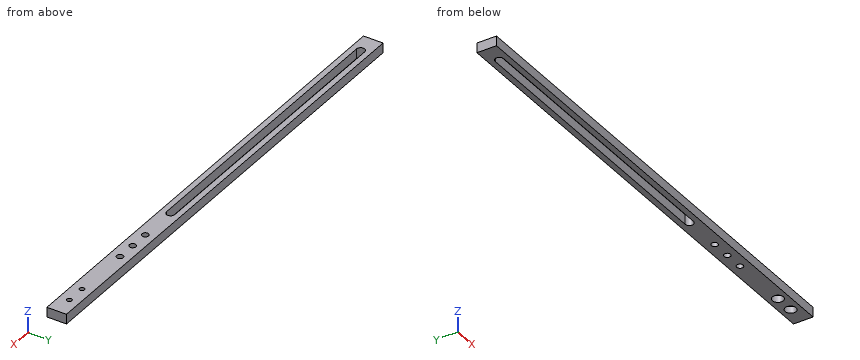
from build123d import *

# Parameters (mm, degrees)
SKETCH_1_W          = 250
SKETCH_1_H          = 10
EXTRUDE_1_DEPTH     = 5
CUT_EXTRUDE_1_DEPTH = 5
SKETCH_3_R          = 1.25
CUT_EXTRUDE_2_DEPTH = 5
SKETCH_4_R          = 2.8
CUT_EXTRUDE_3_DEPTH = 3.5
SKETCH_5_R          = 1.65
CUT_EXTRUDE_4_DEPTH = 10


with BuildPart() as part:
    # Эскиз1 → Бобышка-Вытянуть1 (new body)
    with BuildSketch(Plane.XY):
        Rectangle(SKETCH_1_W, SKETCH_1_H)
    extrude(amount=EXTRUDE_1_DEPTH)

    # Эскиз2 → Вырез-Вытянуть1 (cut)
    with BuildSketch(Plane(origin=(0, 0, 0), x_dir=(-1, 0, 0), z_dir=(0, 0, -1))):
        with BuildLine():
            Line((-35, 2.1), (115, 2.1))
            ThreePointArc((115, 2.1), (117.1, 0), (115, -2.1))
            Line((115, -2.1), (-35, -2.1))
            ThreePointArc((-35, -2.1), (-37.1, 0), (-35, 2.1))
        make_face()
    extrude(amount=-CUT_EXTRUDE_1_DEPTH, mode=Mode.SUBTRACT)

    # Эскиз3 → Вырез-Вытянуть2 (cut)
    with BuildSketch(Plane(origin=(0, 0, 0), x_dir=(-1, 0, 0), z_dir=(0, 0, -1))):
        with Locations((-115, 0)):
            Circle(SKETCH_3_R)
        with Locations((-105, 0)):
            Circle(SKETCH_3_R)
    extrude(amount=-CUT_EXTRUDE_2_DEPTH, mode=Mode.SUBTRACT)

    # Эскиз4 → Вырез-Вытянуть3 (cut)
    with BuildSketch(Plane(origin=(0, 0, 0), x_dir=(-1, 0, 0), z_dir=(0, 0, -1))):
        with Locations((-115, 0)):
            Circle(SKETCH_4_R)
        with Locations((-105, 0)):
            Circle(SKETCH_4_R)
    extrude(amount=-CUT_EXTRUDE_3_DEPTH, mode=Mode.SUBTRACT)

    # Эскиз5 → Вырез-Вытянуть4 (cut)
    with BuildSketch(Plane(origin=(0, 0, 0), x_dir=(-1, 0, 0), z_dir=(0, 0, -1))):
        with Locations((-75, 0)):
            Circle(SKETCH_5_R)
        with Locations((-65, 0)):
            Circle(SKETCH_5_R)
        with Locations((-55, 0)):
            Circle(SKETCH_5_R)
    extrude(amount=-CUT_EXTRUDE_4_DEPTH, mode=Mode.SUBTRACT)


solid = part.part
Read the model definition and answer for the solid it produces. Units are mm, in the model's axes. Give positions to 0.01 mm unless a question says otherwise; leave off trailing zeros. Loops run counter-clockwise (first coordinate to the right, second up) from the corner with the lowest first, then second, coordinate; pieces in that order, holes last. Notation, with made-up numbers: (-23.75, -3.75) -> (-12.75, -3.75) arc R27 ccw to (-12.75, 33.25) -> close; hole circle Ø7 at (0, 75). An arc over 180 degrees is marked (long way). Answer as CSV lines item,"result".
Item 1: This flat-tipped pin is pushed along its axis until it touches: pin 1 (3 mm diameter, centred on x = 104, y = -0.5, fed in from -Z). Where does it stop, or does it pass through?
Returned:
pin 1,"stops at z = 3.5"
Item 2: Find section A-A on x = -44.5. Give the vertices of the cut face in (y, z), plus the area to 3 significant figures.
Returned:
outline,"(-5, 0) -> (-2.1, 0) -> (-2.1, 5) -> (-5, 5) -> close; (2.1, 0) -> (5, 0) -> (5, 5) -> (2.1, 5) -> close"
area,"29.0 mm²"
Item 3: Find section B-B on z = 1.45. Give the vertices of the cut face in (x, y), plus the area to 3 significant figures.
Returned:
outline,"(-125, -5) -> (125, -5) -> (125, 5) -> (-125, 5) -> close; hole (-115, -2.1) -> (35, -2.1) arc R2.1 ccw to (35, 2.1) -> (-115, 2.1) arc R2.1 ccw to start; hole circle Ø3.3 at (55, 0); hole circle Ø3.3 at (65, 0); hole circle Ø3.3 at (75, 0); hole circle Ø5.6 at (105, 0); hole circle Ø5.6 at (115, 0)"
area,"1,780 mm²"
Item 4: Consider line 1 (Y direction, x = 115, z = 2.45); line 2 (Y direction, x = -39, z = 1.05); line 3 (X direction, y = 2.25, z = 1.2). Determine where each line is inside the solid, lowest interval first. Write a range as [from, to].
Returned:
line 1,"y = [-5, -2.8], [2.8, 5]"
line 2,"y = [-5, -2.1], [2.1, 5]"
line 3,"x = [-125, 103.33], [106.67, 113.33], [116.67, 125]"
